Autodesk Inventor part; units mm, degrees
ref_plane "YZ Plane" through (0, 0, 0) normal (1, 0, 0) x (0, 1, 0)
ref_plane "XZ Plane" through (0, 0, 0) normal (0, 1, 0) x (-1, 0, 0)
ref_plane "XY Plane" through (0, 0, 0) normal (0, 0, 1) x (1, 0, 0)
sketch "Sketch1" plane through (0, 0, 0) normal (0, 0, 1) x (1, 0, 0)
  circle A0 centre (0, 0) radius 9.96
  circle A1 centre (0, 45) radius 9.96
  line L0 (-9.96, 45) -> (-9.96, 0)
  line L1 (9.96, 45) -> (9.96, 0)
  dimension "d0" = 19.92
  dimension "d1" = 45
extrude "Plate1" add sketch "Sketch1" along normal blind 1.5
sketch "Sketch2" plane through (0, 0, 1.5) normal (0, 0, 1) x (1, 0, 0)
  circle A0 centre (-7, 0) radius 0.7835
  circle A1 centre (7, 0) radius 0.7835
  circle A2 centre (0, 7) radius 0.7835
  circle A3 centre (0, -7) radius 0.7835
  line L0 (-9.96, 0) -> (-9.96, 45) construction
  line L1 (9.96, 45) -> (9.96, 0) construction
  line L2 (-9.96, 22.5) -> (9.96, 22.5) construction
  point P0 (0, 0)
  point P1 (-7, 45)
  point P2 (7, 45)
  point P3 (0, 38)
  point P4 (0, 52)
hole "Hole1" at (0, 52, 1.5) at (-7, 45, 1.5) at (0, 38, 1.5) at (7, 45, 1.5) at (0, 7, 1.5) at (-7, 0, 1.5) at (0, -7, 1.5) at (7, 0, 1.5) direction (0, 0, -1) diameter 2.1 end through all
sketch "Sketch3" plane through (0, 0, 1.5) normal (0, 0, 1) x (1, 0, 0)
  circle A0 centre (0, 0) radius 1.75
  circle A1 centre (0, 0) radius 2.6
  line L0 (-9.96, 0) -> (-9.96, 45) construction
  line L1 (9.96, 45) -> (9.96, 0) construction
  line L2 (-9.96, 22.5) -> (9.96, 22.5) construction
  circle A2 centre (0, 45) radius 2.6
  point P0 (0, 0)
  dimension "d10" = 5.2
extrude "Extrusion1" cut sketch "Sketch3" against normal through all contours A0 | A1 | A2
sketch "Sketch4" plane through (0, 0, 1.5) normal (0, 0, 1) x (1, 0, 0)
  circle A0 centre (5.865, 29.0135) radius 0.7835
  circle A1 centre (-6.135, 29.0135) radius 0.7835
  circle A2 centre (5.865, 17.1265) radius 0.7835
  circle A3 centre (-6.135, 17.1265) radius 0.7835
  point P0 (0, 0)
hole "Hole2" at (-6.135, 29.0135, 1.5) at (5.865, 29.0135, 1.5) at (-6.135, 17.1265, 1.5) at (5.865, 17.1265, 1.5) direction (0, 0, -1) diameter 2.1 end through all
equation "\"d8\" = Thickness"
equation "\"d18\" = Thickness"
equation "\"d2\" = Thickness"
equation "\"BendReliefWidth\" = Thickness"
equation "\"BendReliefDepth\" = 0.5 * Thickness"
equation "\"CornerReliefSize\" = 4 * Thickness"
equation "\"MinimumRemnant\" = 2 * Thickness"
equation "\"TransitionRadius\" = BendRadius"
equation "\"JacobiRadiusSize\" = BendRadius"
equation "\"GapSize\" = Thickness"
properties part number "axis_3_bottom_frame(top)" material "Aluminum 6061-AHC"
The model under review builds one solid part; all positions refer to its coordinate system, in mm. Round coordinates to 2 decimals unless told otherwise and drop trailing zeros. Write each loop counter-clockwise with the first axis right and the second up, starting at its lowest first coordinate (ties: lowest second). Pieces come first, ordered by that corner, then holes. Notation, with made-up numbers: (75.25, 33.5) -> (129.25, 33.5) arc R8 ccw to (129.25, 47.5) -> close; hole circle Ø9 at (34.25, 45). An arc over 180 degrees is marked (long way). Use CSV: the item, a comma, the result in double quotes.
Q1. Consider section C-C (z = 0.7). State how many separate pieces and enclosed holes the cut face has, then the cut area to 3 significant figures.
Checks:
separate pieces,"1"
enclosed holes,"14"
area,"1,120 mm²"
Q2. Consider section D-D (y = 43). Give the boundary of the cut face in (x, z).
Checks:
outline,"(-9.96, 0) -> (-1.66, 0) -> (-1.66, 1.5) -> (-9.96, 1.5) -> close; (1.66, 0) -> (9.96, 0) -> (9.96, 1.5) -> (1.66, 1.5) -> close"
Q3. Mouldability with a two-part tool opening along X and no side actions: class faces 1 (the flat face through (9.96, 23, 1)), 2 (the cylindrical face through (-0.05, 8.05, 0.74)), 3 (the flat face through (0, 23, 1.5)) as released by +X, released by -X, zero draft, split by the parting line, or undercut.
Checks:
face 1,"released by +X"
face 2,"undercut"
face 3,"zero draft"
Q4. Consider section A-A (y = 7). Give the boundary of the cut face in (x, z), then the cut area to 3 significant figures.
Checks:
outline,"(-9.96, 0) -> (-1.05, 0) -> (-1.05, 1.5) -> (-9.96, 1.5) -> close; (1.05, 0) -> (9.96, 0) -> (9.96, 1.5) -> (1.05, 1.5) -> close"
area,"26.7 mm²"
Q5. To check wall thickness, follow probe 1 along X at (y, z) = (38, 0.6); probe 2 along Y at (x, z) = (1.75, 0.7); probe 3 along Y at (x, z) = (-7, 0.4). State the ranges of each line that lie inside material, in increasing order. Write a range as [from, to].
Checks:
probe 1,"[-9.96, -1.05], [1.05, 9.96]"
probe 2,"[-9.81, -1.92], [1.92, 43.08], [46.92, 54.81]"
probe 3,"[-7.09, -1.05], [1.05, 16.53], [17.72, 28.42], [29.61, 43.95], [46.05, 52.09]"
Q6. Consider section B-B (x = 1.75). Give the boundary of the cut face in (y, z), then the cut area to 3 significant figures.
Checks:
outline,"(-9.81, 0) -> (-1.92, 0) -> (-1.92, 1.5) -> (-9.81, 1.5) -> close; (1.92, 0) -> (43.08, 0) -> (43.08, 1.5) -> (1.92, 1.5) -> close; (46.92, 0) -> (54.81, 0) -> (54.81, 1.5) -> (46.92, 1.5) -> close"
area,"85.4 mm²"
